Can you work these out from the model? Positions are in its coordinate system, mm. A direction names the side the tool comes from. Round coordinates to 2 decimals unless told otherwise and drop trailing zeros. Order: outer loops, then holes, each group sorted by start corner. A loop starts at its lowest first (then second) coordinate and runs counter-clockwise, first axis right, second up. Notation, with made-up numbers: M 63.5,52 L 78.5,52 A8 cw 78.5,59 Z; hole C 45.5,22.5 d2. An arc over 180 degrees is marked long. Answer as a JSON object with one key per item and string values. Group by question number.
from build123d import *

# Parameters (mm, degrees)
SKETCH_W        = 53
SKETCH_H        = 89
PAD_DEPTH       = 2
SKETCH001_W     = 51
SKETCH001_H     = 71
POCKET_DEPTH    = 2
SKETCH002_W     = 53
SKETCH002_H     = 89
SKETCH002_W_2   = 51
SKETCH002_H_2   = 87
PAD001_DEPTH    = 33
SKETCH003_R     = 1.5
PAD002_DEPTH    = 2
PAD003_DEPTH    = 2
POCKET001_DEPTH = 88


with BuildPart() as part:
    # Sketch → Pad (new body)
    with BuildSketch(Plane.XY):
        with Locations((26.5, 44.5)):
            Rectangle(SKETCH_W, SKETCH_H)
    extrude(amount=PAD_DEPTH)

    # Sketch001 (on Face6 of Pad) → Pocket (cut)
    with BuildSketch(Plane.XY.offset(2)):
        with Locations((26.5, 46.5)):
            Rectangle(SKETCH001_W, SKETCH001_H)
    extrude(amount=-POCKET_DEPTH, mode=Mode.SUBTRACT)

    # Sketch002 (on Face5 of Pocket) → Pad001 (join)
    with BuildSketch(Plane.XY.offset(2)):
        with Locations((26.5, 44.5)):
            Rectangle(SKETCH002_W, SKETCH002_H)
        with Locations((26.5, 44.5)):
            Rectangle(SKETCH002_W_2, SKETCH002_H_2, mode=Mode.SUBTRACT)
    extrude(amount=PAD001_DEPTH)

    # Sketch003 (on Face15 of Pad001) → Pad002 (join)
    with BuildSketch(Plane.XY.offset(2)):
        with BuildLine():
            ThreePointArc((4, 82), (6.12132, 82.87868), (7, 85))
            Line((7, 88), (7, 85))
            Line((1, 88), (7, 88))
            Line((1, 82), (1, 88))
            Line((4, 82), (1, 82))
        make_face()
        with Locations((4, 85)):
            Circle(SKETCH003_R, mode=Mode.SUBTRACT)
        with BuildLine():
            ThreePointArc((46, 85), (46.87868, 82.87868), (49, 82))
            Line((52, 82), (49, 82))
            Line((52, 88), (52, 82))
            Line((46, 88), (52, 88))
            Line((46, 85), (46, 88))
        make_face()
        with Locations((49, 85)):
            Circle(SKETCH003_R, mode=Mode.SUBTRACT)
        with BuildLine():
            ThreePointArc((49, 11), (46, 8), (49, 5))
            Line((52, 5), (49, 5))
            Line((52, 11), (52, 5))
            Line((49, 11), (52, 11))
        make_face()
        with Locations((49, 8)):
            Circle(SKETCH003_R, mode=Mode.SUBTRACT)
        with BuildLine():
            ThreePointArc((4, 5), (7, 8), (4, 11))
            Line((1, 11), (4, 11))
            Line((1, 5), (1, 11))
            Line((4, 5), (1, 5))
        make_face()
        with Locations((4, 8)):
            Circle(SKETCH003_R, mode=Mode.SUBTRACT)
    extrude(amount=PAD002_DEPTH)

    # Sketch004 (on Face13 of Pad002) → Pad003 (join)
    with BuildSketch(Plane.XY.offset(35)):
        Polygon((0, 0), (0, 89), (1, 89), (1, 1), (52, 1), (52, 89), (53, 89), (53, 0), align=None)
    extrude(amount=PAD003_DEPTH)

    # Sketch005 (on Face28 of Pad003) → Pocket001 (cut)
    with BuildSketch(Plane(origin=(0, 89, 0), x_dir=(-1, 0, 0), z_dir=(0, 1, 0))):
        Polygon((-52.6, 35), (-52, 37), (-52, 35), align=None)
        Polygon((-1, 35), (-1, 37), (-0.4, 35), align=None)
    extrude(amount=-POCKET001_DEPTH, mode=Mode.SUBTRACT)


solid = part.part
Item 1: Suppose I cut it at B-B, the plane z = 3. Write out the boundary of the cut face in (x, y), and give its area (3 significant figures).
Item 2: Suppose I cut it at D-D, the plane y = 49.5. Write out the boundary of the cut face in (x, z).
Item 3: If we mould it in two halves opening along Y, with no side actions, what happens to faces 3 (the face through (26, 89, 18)), 4 (the face through (53, 45, 18)), 5 (the face through (3.805, 86.487, 2.986))? For each: +Y half, -Y half, draft (parallel to the pull), parting line (faces both ways), or undercut.
Item 4: On a 3-axis mill with a long thin cutter (end or side, diameter ignored), from which of +Z, -Z, +X, -X, +Y, -Y can I reach the whole of each face in a straight line? I mean faces 1 (the face through (1, 45, 17)), 2 (the face through (0, 44, 18)). Say none if no direction works.
Item 5: Suppose I cut it at C-C, the plane z = 24.5. Write out the boundary of the cut face in (x, y), and give its area (3 significant figures).
Item 6: I'm going to push flat-ended pins straight in: pin 1 Ø1.8 at (x, y) = (48, 8.5) entering from +Z; pin 2 Ø2.5 at (x, y) = (4, 85) entering from +Z. Where does each tip first touch, or does it pass through?
Item 7: I need wall thicknesses on line 1 (X direction, y = 85, z = 2.9); line 2 (Y direction, x = 4, z = 2.8); line 3 (Y direction, x = 46, z = 26). Which ranges of each line are inside material? Lowest first, please.
Item 8: Suppose I cut it at A-A, the plane x = 15. Write out the boundary of the cut face in (y, z).
Computed:
{
 "1": {"outline": "M 0,0 L 53,0 L 53,89 L 0,89 Z; hole M 1,1 L 52,1 L 52,5 L 49,5 A3 cw 49,11 L 52,11 L 52,82 L 49,82 A3 cw 46,85 L 46,88 L 7,88 L 7,85 A3 cw 4,82 L 1,82 L 1,11 L 4,11 A3 cw 4,5 L 1,5 Z; hole C 4,8 d3; hole C 4,85 d3; hole C 49,8 d3; hole C 49,85 d3", "area": "384 mm^2"},
 "2": {"outline": "M 0,0 L 1,0 L 1,35 L 0.4,35 L 1,37 L 0,37 Z; M 52,0 L 53,0 L 53,37 L 52,37 L 52.6,35 L 52,35 Z"},
 "3": {"face 3": "+Y half", "face 4": "draft", "face 5": "undercut"},
 "4": {"face 1": "+Z", "face 2": "+Z, -Z, -X, +Y, -Y"},
 "5": {"outline": "M 0,0 L 53,0 L 53,89 L 0,89 Z; hole M 1,1 L 52,1 L 52,88 L 1,88 Z", "area": "280 mm^2"},
 "6": {"pin 1": "stops at z = 4", "pin 2": "stops at z = 2"},
 "7": {"line 1": "x = 0 to 2.5, 5.5 to 7, 46 to 47.5, 50.5 to 53", "line 2": "y = 0 to 1, 5 to 6.5, 9.5 to 11, 82 to 83.5, 86.5 to 89", "line 3": "y = 0 to 1, 88 to 89"},
 "8": {"outline": "M 0,0 L 11,0 L 11,2 L 1,2 L 1,37 L 0,37 Z; M 82,0 L 89,0 L 89,35 L 88,35 L 88,2 L 82,2 Z"}
}
